Read the model definition and answer for the solid it produces. Units are mm, in the model's axes. Face numbers are marked on the shaded views. Give positions to 0.01 mm unless a question says otherwise; leave off trailing zeros. Write each loop counter-clockwise with the first axis right and the second up, starting at its lowest first coordinate (ties: lowest second). Pieces come first, ordered by that corner, then holes. Notation, with made-up numbers: M 76,9 L 88,9 A20 ccw 88,20 Z; hole C -35,77 d7. An arc over 180 degrees is marked long. Put each result on its own line as item: value.
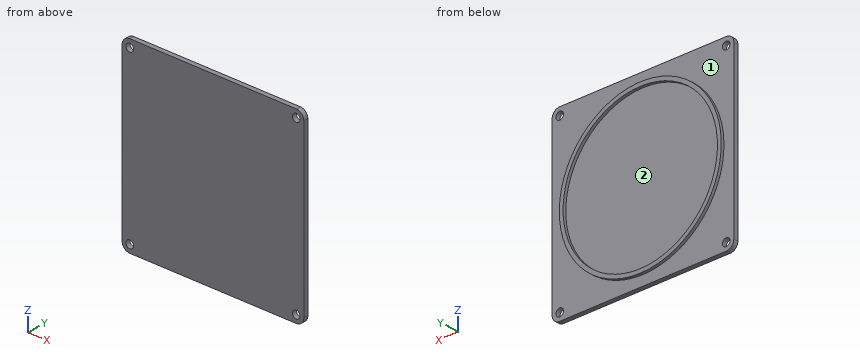
from build123d import *

# Parameters (mm, degrees)
SKETCH1_W           = 120
SKETCH1_H           = 120
BOSS_EXTRUDE1_DEPTH = 3
SKETCH2_R           = 53.5
SKETCH2_R_2         = 51
BOSS_EXTRUDE2_DEPTH = 2
SKETCH3_R           = 2.5
CUT_EXTRUDE1_DEPTH  = 3
FILLET2_R           = 5


with BuildPart() as part:
    # Sketch1 → Boss-Extrude1 (new body)
    with BuildSketch(Plane(origin=(0, 0, 0), x_dir=(1, 0, 0), z_dir=(0, 1, 0))):
        Rectangle(SKETCH1_W, SKETCH1_H)
    extrude(amount=BOSS_EXTRUDE1_DEPTH)

    # Sketch2 → Boss-Extrude2 (add)
    with BuildSketch(Plane(origin=(0, 3, 0), x_dir=(1, 0, 0), z_dir=(0, 1, 0))):
        with Locations(Location((0, 0, 0), (0, 0, 90))):
            Circle(SKETCH2_R)
        with Locations(Location((0, 0, 0), (0, 0, 270))):
            Circle(SKETCH2_R_2, mode=Mode.SUBTRACT)
    extrude(amount=BOSS_EXTRUDE2_DEPTH)

    # Sketch3 → Cut-Extrude1 (cut)
    with BuildSketch(Plane(origin=(0, 3, 0), x_dir=(1, 0, 0), z_dir=(0, 1, 0))):
        with Locations(Location((-55, 55, 0), (0, 0, 270))):
            Circle(SKETCH3_R)
        with Locations(Location((55, 55, 0), (0, 0, 90))):
            Circle(SKETCH3_R)
        with Locations(Location((-55, -55, 0), (0, 0, 90))):
            Circle(SKETCH3_R)
        with Locations(Location((55, -55, 0), (0, 0, 270))):
            Circle(SKETCH3_R)
    extrude(amount=-CUT_EXTRUDE1_DEPTH, mode=Mode.SUBTRACT)

    # Fillet2
    fillet2_edges = [part.edges().sort_by_distance(p)[0] for p in [
        (60, 1.5, 60),
        (-60, 1.5, 60),
        (-60, 1.5, -60),
        (60, 1.5, -60),
    ]]
    fillet(fillet2_edges, radius=FILLET2_R)


solid = part.part
(1) Section A-A on x = 0 is taken. Determine the outline of the cut face in (y, z).
Result:
outline: M 0,-60 L 3,-60 L 3,-53.5 L 5,-53.5 L 5,-51 L 3,-51 L 3,51 L 5,51 L 5,53.5 L 3,53.5 L 3,60 L 0,60 Z
(2) For a pull along Z with two mould halves and no side action, classify the marked faces 1 and 2 as +Z half, -Z half, draft (parallel to the pull), parting line (faces both ways), or undercut.
Result:
face 1: draft
face 2: undercut
(3) Straight lines are drawn through the part: line 1 along X through (y, z) = (1.3, 55); line 2 along X through (y, z) = (4, 0); line 3 along Y through (x, z) = (5, -21). For each, find the intervals that lie inside material, in ascending order. Write a range as from..to.
Result:
line 1: x = -60..-57.5, -52.5..52.5, 57.5..60
line 2: x = -53.5..-51, 51..53.5
line 3: y = 0..3
(4) Given pin 1 Ø4 at (x, z) = (-29, 26) entering from +Y; pin 2 Ø12 at (x, z) = (41, -41.5) entering from +Y, each flat-ended and moving along its own axis, determine where each tip first touches the part or whether it passes through.
Result:
pin 1: stops at y = 3
pin 2: stops at y = 5
(5) Section B-B on z = -17.5 is taken. Determine the outline of the cut face in (x, y).
Result:
outline: M -60,0 L 60,0 L 60,3 L 50.56,3 L 50.56,5 L 47.9,5 L 47.9,3 L -47.9,3 L -47.9,5 L -50.56,5 L -50.56,3 L -60,3 Z
